Model file for the job. Use its own axes, mm. Give positions to 0.01 mm unless a question says otherwise; leave off trailing zeros. Loops run counter-clockwise (first coordinate to the right, second up) from the corner with the lowest first, then second, coordinate; pieces in that order, holes last. Notation, with made-up numbers: M 42,80.25 L 70,80.25 A18 ccw 70,89.25 Z; hole C -23,45.5 d4. An arc over 180 degrees is marked long. Answer in a Markdown table with one row per item.
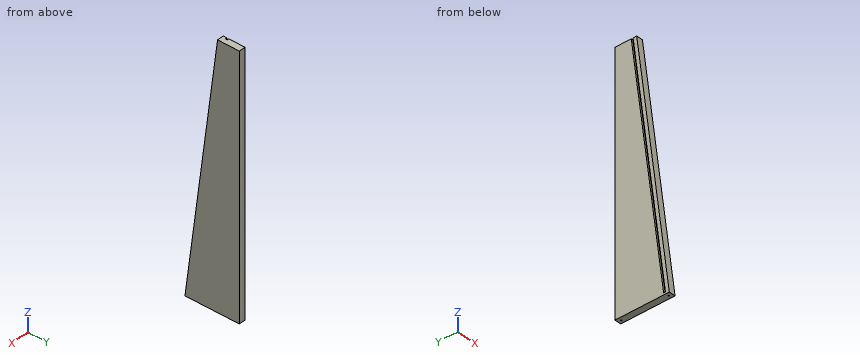
```python
from build123d import *

# Parameters (mm, degrees)
F1_DEPTH = 18
F3_DEPTH = 5
F4_R     = 1.5
F5_DEPTH = 5


with BuildPart() as f1:
    # F0 (on Right) → F1 (new body)
    with BuildSketch(Plane.YZ):
        Polygon((90, 700), (0, 0), (150, 0), (150, 700), align=None)
    extrude(amount=F1_DEPTH)

    # F2 (on face) → F3 (cut)
    with BuildSketch(Plane(origin=(0, 0, 0), x_dir=(0, -1, 0), z_dir=(-1, 0, 0))):
        Polygon((-15.642857, 5), (-10.642857, 5), (-100, 700), (-105, 700), align=None)
    extrude(amount=-F3_DEPTH, mode=Mode.SUBTRACT)

    # F4 (on face) → F5 (cut)
    with BuildSketch(Plane(origin=(0, 0, 0), x_dir=(1, 0, 0), z_dir=(0, 0, -1))):
        with Locations((9, -10)):
            Circle(F4_R)
        with Locations((9, -140)):
            Circle(F4_R)
    extrude(amount=-F5_DEPTH, mode=Mode.SUBTRACT)


solid = f1.part
```
(1) Wall check: L1, parallel to X at y = 140, z = 1.25; L2, parallel to Y at x = 9, z = 3.55; L3, parallel to Y at x = 9, z = 3. Give the ranges that are in metal, low to high.
Established:
| item | result |
|---|---|
| L1 | x = 0 to 7.5, 10.5 to 18 |
| L2 | y = 0.46 to 8.5, 11.5 to 138.5, 141.5 to 150 |
| L3 | y = 0.39 to 8.5, 11.5 to 138.5, 141.5 to 150 |
(2) Saw through at B-B, the plane z = 310.5. Give the cut face in (x, y), and give its area (3 significant figures).
Established:
| item | result |
|---|---|
| outline | M 0,39.92 L 18,39.92 L 18,150 L 0,150 L 0,54.92 L 5,54.92 L 5,49.92 L 0,49.92 Z |
| area | 1,960 mm2 |
(3) Flat gauge pins, fed straight in: P1, Ø10, axis at x = 13, z = 502, coming from the -Y side; P2, Ø2.5, axis at x = 9, y = 10, coming from the -Z side. Where does each tip first touch, or does it go through?
Established:
| item | result |
|---|---|
| P1 | stops at y = 63.9 |
| P2 | stops at z = 5 |
(4) Saw through at A-A, the plane y = 80. Give the cut face in (x, z), and give its area (3 significant figures).
Established:
| item | result |
|---|---|
| outline | M 0,0 L 18,0 L 18,622.22 L 0,622.22 L 0,544.44 L 5,544.44 L 5,505.56 L 0,505.56 Z |
| area | 11,000 mm2 |
